Could you check a few things on this model? Use its own coordinates, in mm. A direction names the side the tool comes from. Round coordinates to 2 decimals unless told otherwise and drop trailing zeros. Order: outer loops, then holes, each group sorted by start corner. A loop starts at its lowest first (then second) coordinate and runs counter-clockwise, first axis right, second up. Notation, with made-up numbers: (4.5, -7.5) -> (23.5, -7.5) arc R13 cw to (23.5, 0.5) -> close; hole circle Ø1 at (81, 47). An arc over 180 degrees is marked (long way). Put each result on its own line as item: value. Start each with the question number.
from build123d import *

# Parameters (mm, degrees)
SKETCH1_W           = 200
SKETCH1_H           = 200
BOSS_EXTRUDE1_DEPTH = 10
SKETCH2_W           = 100
SKETCH2_H           = 100
BOSS_EXTRUDE2_DEPTH = 420
SKETCH3_R           = 40
CUT_EXTRUDE1_DEPTH  = 420
BOSS_EXTRUDE4_START = 100
SKETCH5_R           = 50
SKETCH5_R_2         = 40
BOSS_EXTRUDE4_DEPTH = 100


with BuildPart() as part:
    # Sketch1 → Boss-Extrude1 (new body)
    with BuildSketch(Plane(origin=(0, 0, 0), x_dir=(1, 0, 0), z_dir=(0, 1, 0))):
        with Locations((100, 100)):
            Rectangle(SKETCH1_W, SKETCH1_H)
    extrude(amount=BOSS_EXTRUDE1_DEPTH)

    # Sketch2 → Boss-Extrude2 (add)
    with BuildSketch(Plane(origin=(0, 10, 0), x_dir=(1, 0, 0), z_dir=(0, 1, 0))):
        with Locations((100, 100)):
            Rectangle(SKETCH2_W, SKETCH2_H)
    extrude(amount=BOSS_EXTRUDE2_DEPTH)

    # Sketch3 → Cut-Extrude1 (cut)
    with BuildSketch(Plane(origin=(0, 430, 0), x_dir=(1, 0, 0), z_dir=(0, 1, 0))):
        with Locations(Location((100, 100, 0), (0, 0, 270))):
            Circle(SKETCH3_R)
    extrude(amount=-CUT_EXTRUDE1_DEPTH, mode=Mode.SUBTRACT)

    # Sketch5 → Boss-Extrude4 (add)
    with BuildSketch(Plane(origin=(0, 430, 0), x_dir=(1, 0, 0), z_dir=(0, 1, 0)).offset(BOSS_EXTRUDE4_START)):
        with Locations(Location((100, 100, 0), (0, 0, 270))):
            Circle(SKETCH5_R)
        with Locations(Location((100, 100, 0), (0, 0, 270))):
            Circle(SKETCH5_R_2, mode=Mode.SUBTRACT)
    extrude(amount=-BOSS_EXTRUDE4_DEPTH)


solid = part.part
1. For pin 1 Ø5 at (x, z) = (57.5, -57.5) entering from +Y; pin 2 Ø2 at (x, y) = (101.5, 54.5) entering from +Z; pin 3 Ø3 at (y, z) = (335, -102.5) entering from +X, each with a flat end and sliding along its axis, tell me the tip position at first contact or that it passes through.
2. Which directions (+Z, -Z, +X, -X, +Y, -Y) give clear straight access to the entire face, cutting with the end or side of a thin tool? Please do faces 1 (the face through (150, 217, -99)), 2 (the face through (60, 430, -138)), 3 (the face through (60, 430, -62)).
3. If we section it at B-B, the plane x = 36: Please give me the cut outline in (y, z).
4. If we section it at D-D, the plane y = 292.5: Please give me the cut outline in (x, z), then the cut area to 3 significant figures.
5. I need wall thicknesses on L1, parallel to X at y = 254.5, z = -100; L2, parallel to X at y = 152, z = -97.5; L3, parallel to Y at x = 14.5, z = -161.5. Which ranges of each line are inside material? Lowest first, please.
6. Thinking about a two-plate mould opening in Z: for faces 4 (the face through (99, 217, -50)), 5 (the face through (112.015, 273.64, -61.847)), 6 (the face through (101, 10, -101)), 7 (the face through (140, 430, -60)), which applies, +Z half, -Z half, draft (parallel to the pull), parting line (faces both ways), or undercut?
7. If we section it at C-C, the plane z = -111.5: Please give me the cut outline in (x, y), then the cut area to 3 significant figures.
8. If we section it at A-A, the plane y = 497: Please give me the cut outline in (x, z).
Results below:
1. pin 1: y = 430
1. pin 2: z = -50
1. pin 3: x = 150
2. face 1: +Z, -Z, +X, +Y
2. face 2: -Z, -X, +Y
2. face 3: +Z, -X, +Y
3. outline: (0, -200) -> (10, -200) -> (10, 0) -> (0, 0) -> close
4. outline: (50, -150) -> (150, -150) -> (150, -50) -> (50, -50) -> close; hole circle Ø80 at (100, -100)
4. area: 4,970 mm2
5. L1: 50 to 60, 140 to 150
5. L2: 50 to 60.08, 139.92 to 150
5. L3: 0 to 10
6. face 4: +Z half
6. face 5: undercut
6. face 6: undercut
6. face 7: draft
7. outline: (0, 0) -> (200, 0) -> (200, 10) -> (150, 10) -> (150, 430) -> (148.66, 430) -> (148.66, 530) -> (138.31, 530) -> (138.31, 10) -> (61.69, 10) -> (61.69, 530) -> (51.34, 530) -> (51.34, 430) -> (50, 430) -> (50, 10) -> (0, 10) -> close
7. area: 13,900 mm2
8. outline: circle Ø100 at (100, -100); hole circle Ø80 at (100, -100)
